Input: part model. Units: mm. Frame: model coordinates. Face numbers are marked on the shaded views. A direction names the side the tool comes from. Coordinates: 2 decimals unless noted, no trailing zeros. Order: outer loops, then holes, each group sorted by start corner. A loop starts at its lowest first (then second) coordinate and runs counter-clockwise, first axis right, second up. Notation, with made-up numbers: M 0,85.5 L 58,85.5 A28 cw 58,112.5 Z; hole C 14,33.5 d8. An arc over 180 degrees is marked long. One line per item, written item: value.
```python
from build123d import *

# Parameters (mm, degrees)
F2_DEPTH = 12.5
F3_R     = 3
F4_DEPTH = 16
F5_SIZE  = 0.5
F6_SIZE  = 0.5


with BuildPart() as f1:
    # F0 (on Front) → F1 (revolve)
    with BuildSketch(Plane.XZ):
        with BuildLine():
            Line((0, 0), (0, 0.9005403525))
            ThreePointArc((0, 0.9005403525), (-5.0170534649, 0.6935333438), (-10, 0.0739195926))
            Line((-10, 0.0739195926), (-10, 0))
            Line((-10, 0), (0, 0))
        make_face()
        with BuildLine():
            ThreePointArc((-10, 0.0739195926), (-5.0170534649, 0.6935333438), (0, 0.9005403525))
            Line((0, 0.9005403525), (0, 5))
            Line((0, 5), (-3.694741217, 5))
            ThreePointArc((-3.694741217, 5), (-4.4495838523, 5.312666057), (-4.7622499093, 6.0675086923))
            Line((-4.7622499093, 6.0675086923), (-4.7622499093, 15.345285621))
            Line((-4.7622499093, 15.345285621), (-4.7622499093, 15.8448135736))
            ThreePointArc((-4.7622499093, 15.8448135736), (-5.6281002444, 21.0608384026), (-8, 25.7863757656))
            Line((-8, 25.7863757656), (-8, 29))
            ThreePointArc((-8, 29), (-8.2928932188, 29.7071067812), (-9, 30))
            Line((-9, 30), (-10, 30))
            Line((-10, 30), (-10, 25.1294640906))
            ThreePointArc((-10, 25.1294640906), (-6.7604826649, 15.5950495973), (-10, 6.0606351041))
            Line((-10, 6.0606351041), (-10, 0.0739195926))
        make_face()
    revolve(axis=Axis((0, 0, 31.9755728546), (0, 0, 1)))

    # F0 (on Front) → F2 (cut, symmetric)
    with BuildSketch(Plane.XZ):
        with BuildLine():
            Line((0, 0), (0, 0.9005403525))
            ThreePointArc((0, 0.9005403525), (-5.0170534649, 0.6935333438), (-10, 0.0739195926))
            Line((-10, 0.0739195926), (-10, 0))
            Line((-10, 0), (0, 0))
        make_face()
        with BuildLine():
            ThreePointArc((10, 0.0739195926), (5.0170534649, 0.6935333438), (0, 0.9005403525))
            Line((0, 0.9005403525), (0, 0))
            Line((0, 0), (10, 0))
            Line((10, 0), (10, 0.0739195926))
        make_face()
    extrude(amount=F2_DEPTH, both=True, mode=Mode.SUBTRACT)

    # F3 (on face) → F4 (join)
    with BuildSketch(Plane.XY.offset(5)):
        Circle(F3_R)
    extrude(amount=-F4_DEPTH)

    # F5
    f5_edges = [f1.edges().sort_by_distance(p)[0] for p in [
        (10, 0, 30),
    ]]
    chamfer(f5_edges, length=F5_SIZE)

    # F6
    f6_edges = [f1.edges().sort_by_distance(p)[0] for p in [
        (-3, 0, -11),
    ]]
    chamfer(f6_edges, length=F6_SIZE)


solid = f1.part
```
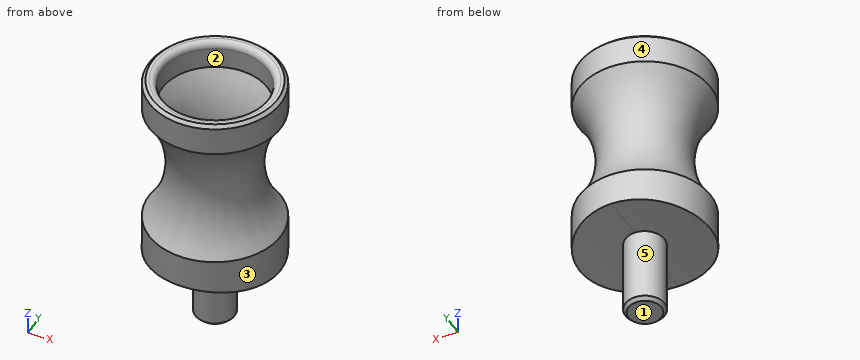
(1) Cut plane C-C on z = 14. Output: boundary loops of the cut face in (x, y), plus the area to 3 significant figures.
Data:
outline: C 0,0 d13.68; hole C 0,0 d9.52
area: 75.8 mm2
(2) Cut plane B-B on y = 0. Output: boundary loops of the cut face in (x, z), plus the area to 3 significant figures.
Data:
outline: M -10,0.07 A60.9 cw -3,0.83 L -3,-10.5 L -2.5,-11 L 2.5,-11 L 3,-10.5 L 3,0.83 A60.9 cw 10,0.07 L 10,6.06 A15.65 cw 10,25.13 L 10,29.5 L 9.5,30 L 9,30 A1 ccw 8,29 L 8,25.79 A17.65 ccw 4.76,15.84 L 4.76,6.07 A1.07 cw 3.69,5 L -3.69,5 A1.07 cw -4.76,6.07 L -4.76,15.84 A17.65 ccw -8,25.79 L -8,29 A1 ccw -9,30 L -9.5,30 L -10,29.5 L -10,25.13 A15.65 cw -10,6.06 Z
area: 288 mm2
(3) Cut plane A-A on z = -2.5. Output: boundary loops of the cut face in (x, y), plus the area to 3 significant figures.
Data:
outline: C 0,0 d6
area: 28.3 mm2
(4) Ray query, line 1 (Y direction, x = 0, z = 26.5); line 2 (Z direction, x = -6.75, y = -7.25); line 3 (Y direction, x = 3.5, z = 18). Return the intervals inside material, ascending. Write a range as from..to.
Data:
line 1: y = -10..-8, 8..10
line 2: z = 0.53..6.18, 25.01..29.59
line 3: y = -6..-3.47, 3.47..6
(5) First-contact query: pin 1 (2 mm diameter, centred on x = -1, y = 0, fed in from +Z); pin 2 (6 mm diameter, centred on y = 7.5, z = 0.5, fed in from +X); pin 3 (3 mm diameter, centred on y = 3.5, z = 8.5, fed in from -X) (3 decimals). Flat tips, straight axial feed; report the tip coordinate or a pass-through.
Data:
pin 1: stops at z = 5
pin 2: stops at x = 8.93
pin 3: stops at x = -8.785
(6) Draft query along X for the marked faces 1, 2 and 3. Return one class per face: released by +X, released by -X, zero draft, split by the parting line, or undercut.
Data:
face 1: zero draft
face 2: undercut
face 3: split by the parting line
(7) Access query for the marked faces 4 and 5. Directions: +Z, -Z, +X, -X, +Y, -Y. A direction counts if a zero-diameter tool reaches every point of the face in a straight line with its end or side. Return the directions, or none.
Data:
face 4: +Z, -Z
face 5: -Z
